Autodesk Inventor part; units mm, degrees
ref_plane "YZ Plane" through (0, 0, 0) normal (1, 0, 0) x (0, 1, 0)
ref_plane "XZ Plane" through (0, 0, 0) normal (0, 1, 0) x (-1, 0, 0)
ref_plane "XY Plane" through (0, 0, 0) normal (0, 0, 1) x (1, 0, 0)
sketch "Boceto1" plane through (0, 0, 0) normal (0, 1, 0) x (-1, 0, 0)
  line L0 (-1.5, -48.5) -> (1.5, -48.5)
  line L1 (1.5, -48.5) -> (1.5, 48.5)
  line L2 (1.5, 48.5) -> (-1.5, 48.5)
  line L3 (-1.5, 48.5) -> (-1.5, -48.5)
  line L4 (-1.5, -48.5) -> (1.5, 48.5) construction
  line L5 (1.5, -48.5) -> (-1.5, 48.5) construction
  point P0 (0, 0)
  dimension "d0" = 3
  dimension "d1" = 97
extrude "Extrusión1" add sketch "Boceto1" along normal blind 180
sketch "Boceto2" plane through (-1.5, 0, -48.5) normal (-1, 0, 0) x (0, 0, 1)
  line L0 (97, 90.5) -> (0, 90.5)
  circle A0 centre (23.1283, 84.5) radius 1.25
  circle A1 centre (73.8717, 84.5) radius 1.25
  line L1 (30.1317, 63.5948) -> (30.1317, 90.5)
  line L2 (66.8717, 90.5) -> (66.8717, 63.5948)
  line L3 (66.8717, 63.5948) -> (30.1317, 63.5948)
  line L4 (30.1317, 63.5948) -> (30.1317, 90.5)
  line L5 (66.8717, 90.5) -> (66.8717, 63.5948)
  point P0 (48.5, 0)
extrude "Extrusión2" cut sketch "Boceto2" against normal through all contours L2 L3 L1 L0
sketch "Boceto3" plane through (-1.5, 0, -48.5) normal (-1, 0, 0) x (0, 0, 1)
  circle A0 centre (6.5, 6.5) radius 1.25
  circle A1 centre (90.5, 6.5) radius 1.25
  circle A2 centre (90.5, 84) radius 1.5
  circle A3 centre (6.5, 84) radius 1.5
  point P0 (48.5, 0)
extrude "Extrusión3" cut sketch "Boceto3" against normal through all
sketch "Boceto4" plane through (-1.5, 0, -48.5) normal (-1, 0, 0) x (0, 0, 1)
  line L0 (80, 148.5) -> (17, 148.5)
  line L1 (0, 148.5) -> (97, 148.5)
  line L2 (6.3714, 170) -> (90.6286, 170)
  line L3 (48.5, 148.5) -> (48.5, 170)
  line L4 (48.5, 159.25) -> (24.25, 159.25)
  line L5 (24.25, 159.25) -> (72.75, 159.25)
  circle A0 centre (24.25, 159.25) radius 1.5
  circle A1 centre (72.75, 159.25) radius 1.5
  point P0 (48.5, 0)
  dimension "d8" = 24.25
  dimension "d9" = 48.5
  dimension "d10" = 3
  dimension "d11" = 3
hole "Agujero1" at (-1.5, 159.25, -24.25) at (-1.5, 159.25, 24.25) direction (1, 0, 0) diameter 3 end through all
properties part number "Panel3"
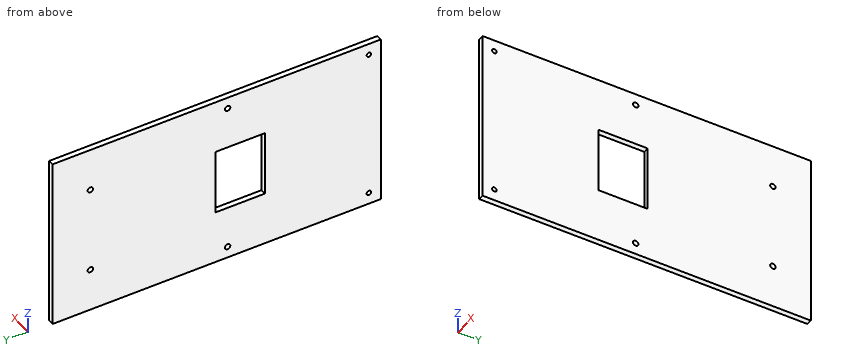
Can you work these out from the model? Positions are in its coordinate system, mm. Round coordinates to 2 decimals unless told otherwise and drop trailing zeros. Write each loop counter-clockwise with the first axis right and the second up, starting at its lowest first coordinate (ties: lowest second). Pieces come first, ordered by that corner, then holes. Notation, with made-up numbers: (2, -3) - (45, -3) arc R26 ccw to (45, 18) - close; hole circle Ø3 at (-39.75, 54). An arc over 180 degrees is marked (long way). Write each question's results on one line, items separated by ' | '. Start each with the question number.
1) For pin 1 Ø1.5 at (y, z) = (6.5, 42) entering from -X, with a flat end and sliding along its axis, tell me the tip position at first contact or that it passes through.
2) Please list where these lines run through material, in increasing order: line 1 (Y direction, x = -0.15, z = -42); line 2 (Z direction, x = 0, y = 159.25); line 3 (Z direction, x = -0.4, y = 84).
3) Suppose I cut it at A-A (x = -0.1). List the corners of the cut face in (y, z) for me.
Here are the results:
1) pin 1: passes through
2) line 1: y = 0 to 5.25, 7.75 to 82.5, 85.5 to 180 | line 2: z = -48.5 to -25.75, -22.75 to 22.75, 25.75 to 48.5 | line 3: z = -48.5 to -43.5, -40.5 to -18.37, 18.37 to 40.5, 43.5 to 48.5
3) outline: (0, -48.5) - (180, -48.5) - (180, 48.5) - (0, 48.5) - close; hole circle Ø2.5 at (6.5, -42); hole circle Ø2.5 at (6.5, 42); hole (63.59, -18.37) - (90.5, -18.37) - (90.5, 18.37) - (63.59, 18.37) - close; hole circle Ø3 at (84, -42); hole circle Ø3 at (84, 42); hole circle Ø3 at (159.25, -24.25); hole circle Ø3 at (159.25, 24.25)
